Could you check a few things on this model? Use its own coordinates, in mm. Coordinates: 2 decimals unless noted, no trailing zeros. One line per item, written item: value. Start each with the question number.
(1) I'm going to push a flat-ended pin straight in: P1, Ø0.6, axis at x = 36.5, z = -2, coming from the +Y side. Where does the tip first touch, or does it pass through?
(2) If I drill on line 1 along Y through (x, z) = (50.5, -2.25), over which ranges is the centre line in solid material (lowest first)? Write a range as from..to.
(3) If we section it at A-A on y = 6.75: Count the separate pieces of the cut face and the enclosed holes in it, then the cut area to 3 significant figures.
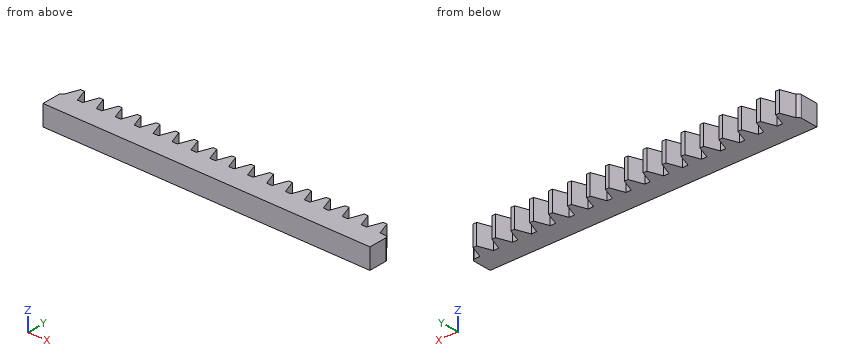
```python
from build123d import *

# Parameters (mm, degrees)
BLANKSKE_W        = 54.3
BLANKSKE_H        = 5.7
BLANK_DEPTH       = 3.4
TOOTHCUTSIM_DEPTH = 55.704113191
TEETHCUTS_COUNT   = 18
TEETHCUTS_PITCH   = 3.14159265
VERRUNDUNG1_R     = 0.5
VERRUNDUNG2_R     = 0.5
SCALE1_SCALE      = 1.46


with BuildPart() as part:
    # BlankSke → Blank (new body)
    with BuildSketch(Plane.XY):
        with Locations((27.15, 2.85)):
            Rectangle(BLANKSKE_W, BLANKSKE_H)
    extrude(amount=-BLANK_DEPTH)

    # TooCutSkeSim → ToothCutSim (cut, through all)
    with BuildSketch(Plane.XY):
        Polygon((0.44443537, 3.45), (-0.44443537, 3.45), (-1.272613241, 5.7254), (1.272613241, 5.7254), align=None)
    toothcutsim = extrude(amount=-TOOTHCUTSIM_DEPTH, mode=Mode.SUBTRACT)

    # TeethCuts: ToothCutSim ×18
    with Locations(*[(i * TEETHCUTS_PITCH, 0, 0) for i in range(1, TEETHCUTS_COUNT)]):
        add(toothcutsim, mode=Mode.SUBTRACT)

    # Verrundung1
    # the kernel refuses this fillet: 0.5 mm, written as the material it takes off along each edge
    with BuildSketch(Plane(origin=(54.3, 4.682214995, -7.723886484), x_dir=(0, -1, 0), z_dir=(0, 0, 1))) as verrundung1_piece_1:
        with BuildLine():
            CenterArc((1.729554594, -0.5), VERRUNDUNG1_R, 90, 84.086849411)
            Line((1.232214995, -0.44848958), (1.222268203, -0.447459372))
            ThreePointArc((1.222268203, -0.447459372), (0.612687296, -0.233641716), (-0.003420201, -0.009396926))
            Line((-0.003420201, -0.009396926), (0, 0.01))
            Line((0, 0.01), (1.729554594, 0.01))
            Line((1.729554594, 0.01), (1.729554594, 0))
        make_face()
    extrude(amount=12.047772969, mode=Mode.SUBTRACT)

    # Verrundung2
    # the kernel refuses this fillet: 0.5 mm, written as the material it takes off along each edge
    with BuildSketch(Plane(origin=(0, 3.45, 1.242257451), x_dir=(0, -1, 0), z_dir=(0, 0, -1))) as verrundung2_piece_1:
        with BuildLine():
            CenterArc((0.49690298, -0.5), VERRUNDUNG2_R, 90, 83.619583418)
            Line((0, -0.44443537), (-0.00993806, -0.443324077))
            ThreePointArc((-0.00993806, -0.443324077), (-0.01, -0.222217685), (-0.01, 0))
            Line((-0.01, 0), (0, 0.01))
            Line((0, 0.01), (0.49690298, 0.01))
            Line((0.49690298, 0.01), (0.49690298, 0))
        make_face()
    extrude(amount=5.884514902, mode=Mode.SUBTRACT)


with BuildPart() as part_1:
    # Scale1: scaled about (0, 0, 0)
    add(part.part.scale(SCALE1_SCALE))


solid = part_1.part
```
Values:
1. P1: stops at y = 5.04
2. line 1: y = 0..5.04
3. separate pieces: 17
3. enclosed holes: 0
3. area: 172 mm2
